The figure shows three views and two pictorial views of one solid part (mm, origin at its lowest corner). Answer the questions. Coordinates: 2 decimals unless noted, no trailing zeros. Order: outer loops, then holes, each group sorted by start corner. A loop starts at its lowest first (then second) coordinate and runs counter-clockwise, first axis right, second up.
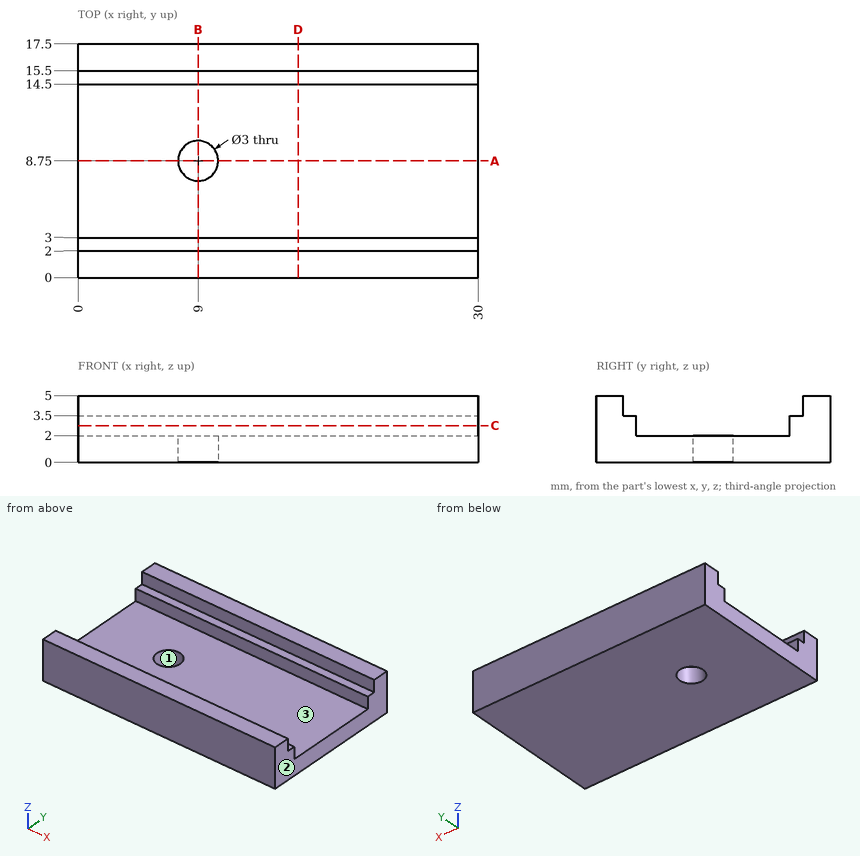
1) The mould has two halves that part along X. Classify the marked faces 1, 2 and 3: released by +X, released by -X, zero draft, split by the parting line, or undercut.
2) A cutting plane is placed at A-A, the plane y = 8.75. Write down the section's boundary in (x, z), plus the area to 3 significant figures.
3) Straight lines are drawn through the part: probe 1 along Y at (x, z) = (8.25, 2.1); probe 2 along Y at (x, z) = (9, 1.1); probe 3 along Z at (x, y) = (25, 11). For each, find the intervals that lie inside material, in ascending order.
4) A cutting plane is placed at B-B, the plane x = 9. Write down the section's boundary in (y, z).
5) A cutting plane is placed at C-C, the plane z = 2.75. Write down the section's boundary in (x, y).
6) Each of these flat-tipped pins is pushed along its axis until it touches: P1, Ø4, axis at x = 13.5, y = 10, coming from the +Z side; P2, Ø0.5, axis at x = 21.5, y = 15, coming from the +Z side. Where does it stop, or does it pass through?
7) A cutting plane is placed at D-D, the plane x = 16.5. Write down the section's boundary in (y, z).
Working result:
1. face 1: undercut
1. face 2: released by +X
1. face 3: zero draft
2. outline: (0, 0) - (7.5, 0) - (7.5, 2) - (0, 2) - close; (10.5, 0) - (30, 0) - (30, 2) - (10.5, 2) - close
2. area: 54.0 mm2
3. probe 1: y = 0 to 3, 14.5 to 17.5
3. probe 2: y = 0 to 7.25, 10.25 to 17.5
3. probe 3: z = 0 to 2
4. outline: (0, 0) - (7.25, 0) - (7.25, 2) - (3, 2) - (3, 3.5) - (2, 3.5) - (2, 5) - (0, 5) - close; (10.25, 0) - (17.5, 0) - (17.5, 5) - (15.5, 5) - (15.5, 3.5) - (14.5, 3.5) - (14.5, 2) - (10.25, 2) - close
5. outline: (0, 0) - (30, 0) - (30, 3) - (0, 3) - close; (0, 14.5) - (30, 14.5) - (30, 17.5) - (0, 17.5) - close
6. P1: stops at z = 2
6. P2: stops at z = 3.5
7. outline: (0, 0) - (17.5, 0) - (17.5, 5) - (15.5, 5) - (15.5, 3.5) - (14.5, 3.5) - (14.5, 2) - (3, 2) - (3, 3.5) - (2, 3.5) - (2, 5) - (0, 5) - close
